Here's how the part is built. I have some questions about the finished solid (model axes, mm). Give positions to 0.01 mm unless a question says otherwise; leave off trailing zeros. Write each loop counter-clockwise with the first axis right and the second up, starting at its lowest first coordinate (ties: lowest second). Pieces come first, ordered by that corner, then holes. Notation, with made-up numbers: M 0,-35 L 46,-35 A35 ccw 46,-2 Z; hole C -18,-34 d6. An arc over 180 degrees is marked long. Answer as CSV lines item,"result". Start each with the question number.
Q1. Suppose I cut it at A-A (x = 40). Write out the boundary of the cut face in (y, z) (3 decimals), then the cut area to 3 significant figures.
Q2. For pin 1 (1 mm diameter, centred on y = 2, z = 30.5, fed in from +X); pin 2 (1 mm diameter, centred on x = -25, y = 0.5, fed in from +Z) (3 decimals); pin 3 (1.6 mm diameter, centred on y = 1.5, z = 51, fed in from +X), each with a flat end and sliding along its axis, tell me the tip position at first contact or that it passes through.
Q3. If I drill on line 1 along X through (y, z) = (2.35, 21.5); line 2 along Z through (x, y) = (14, 1.4) (3 decimals), over which ranges is the centre line in solid material (lowest first)?
Q4. Suppose I cut it at B-B (z = -19). Write out the boundary of the cut face in (x, y) (3 decimals).
```python
from build123d import *

# Parameters (mm, degrees)
SKETCH1_W               = 101.6
SKETCH1_H               = 107.95
BOSS_EXTRUDE1_DEPTH     = 3.175
CUT_EXTRUDE1_DEPTH      = 75.189091179
CUT_EXTRUDE1_DEPTH_BACK = 75.189091179
SKETCH2_W               = 3.429
SKETCH2_H               = 6.604


with BuildPart() as part:
    # Sketch1 → Boss-Extrude1 (new body)
    with BuildSketch(Plane(origin=(0, 0, 0), x_dir=(1, 0, 0), z_dir=(0, 1, 0))):
        Rectangle(SKETCH1_W, SKETCH1_H)
    extrude(amount=BOSS_EXTRUDE1_DEPTH)

    # Sketch2 → Cut-Extrude1 (cut, two sides: drawn at the far end of the back side and taken through both)
    with BuildSketch(Plane(origin=(0, 3.175, 0), x_dir=(1, 0, 0), z_dir=(0, 1, 0)).offset(-CUT_EXTRUDE1_DEPTH_BACK)):
        Polygon((22.098, -47.625), (28.194, -47.625), (28.194, -54.229), (34.798, -54.229), (34.798, -47.625), (47.371, -47.625), (47.371, -41.021), (50.8, -41.021), (50.8, -47.625), (50.8, -92.544961432), (-50.8, -92.544961432), (-50.8, -47.625), (-50.8, -41.021), (-47.371, -41.021), (-47.371, -47.625), (-35.306, -47.625), (-35.306, -54.229), (-28.702, -54.229), (-28.702, -47.625), (-22.606, -47.625), (-22.606, -54.229), (-16.002, -54.229), (-16.002, -47.625), (-9.906, -47.625), (-9.906, -54.229), (-3.302, -54.229), (-3.302, -47.625), (2.794, -47.625), (2.794, -54.229), (9.398, -54.229), (9.398, -47.625), (15.494, -47.625), (15.494, -54.229), (22.098, -54.229), align=None)
        with Locations((-49.0855, 31.75)):
            Rectangle(SKETCH2_W, SKETCH2_H)
        with Locations((-49.0855, 19.177)):
            Rectangle(SKETCH2_W, SKETCH2_H)
        with Locations((-49.0855, 6.477)):
            Rectangle(SKETCH2_W, SKETCH2_H)
        with Locations((-49.0855, -6.223)):
            Rectangle(SKETCH2_W, SKETCH2_H)
        with Locations((-49.0855, -18.923)):
            Rectangle(SKETCH2_W, SKETCH2_H)
        with Locations((-49.0855, -31.623)):
            Rectangle(SKETCH2_W, SKETCH2_H)
        with Locations((49.0855, -31.623)):
            Rectangle(SKETCH2_W, SKETCH2_H)
        with Locations((49.0855, -18.923)):
            Rectangle(SKETCH2_W, SKETCH2_H)
        with Locations((49.0855, -6.223)):
            Rectangle(SKETCH2_W, SKETCH2_H)
        with Locations((49.0855, 6.477)):
            Rectangle(SKETCH2_W, SKETCH2_H)
        with Locations((49.0855, 19.177)):
            Rectangle(SKETCH2_W, SKETCH2_H)
        with Locations((49.0855, 31.75)):
            Rectangle(SKETCH2_W, SKETCH2_H)
        with Locations((49.0855, 44.45)):
            Rectangle(SKETCH2_W, SKETCH2_H)
        with Locations((-49.0855, 44.45)):
            Rectangle(SKETCH2_W, SKETCH2_H)
    extrude(amount=CUT_EXTRUDE1_DEPTH + CUT_EXTRUDE1_DEPTH_BACK, mode=Mode.SUBTRACT)


solid = part.part
```
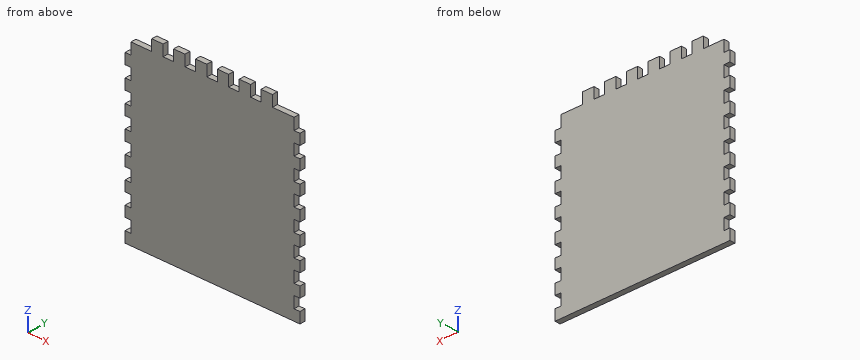
Resolved:
1,outline,"M 0,-53.975 L 3.175,-53.975 L 3.175,47.625 L 0,47.625 Z"
1,area,"323 mm^2"
2,pin 1,"x = 47.37"
2,pin 2,"z = 47.625"
2,pin 3,"x = 34.8"
3,line 1,"-47.37 to 47.37"
3,line 2,"-53.975 to 47.625"
4,outline,"M -47.371,0 L 47.371,0 L 47.371,3.175 L -47.371,3.175 Z"
